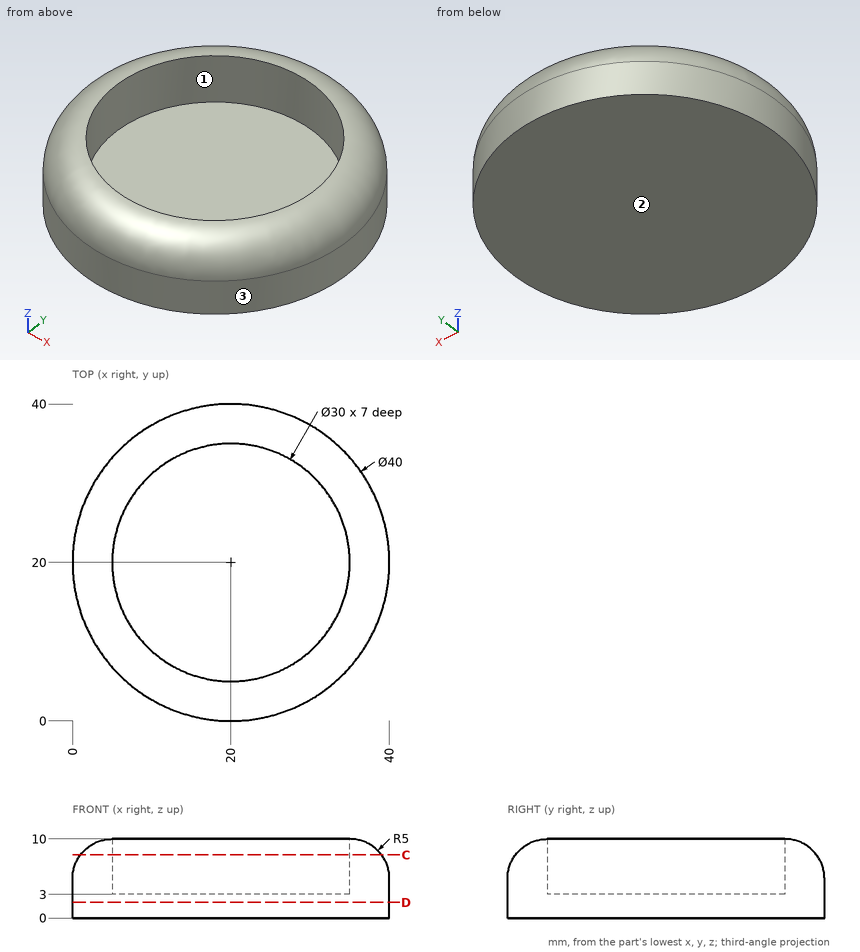
Design review of the part shown in the three views and the two pictorial views. Dimensions are in mm from the part's minimum x, y and z. Give positions to 0.01 mm unless a question says otherwise; leave off trailing zeros. Loops run counter-clockwise (first coordinate to the right, second up) from the corner with the lowest first, then second, coordinate; pieces in that order, holes last. Notation, with made-up numbers: (74.25, 55) -> (89.25, 55) arc R31 cw to (89.25, 85) -> close; hole circle Ø8 at (7.5, -25.75). An arc over 180 degrees is marked (long way). One line per question, with ' | ' between items.
1) To check wall thickness, follow probe 1 along Y at (x, z) = (20, 5); probe 2 along Z at (x, y) = (23, 32.5); probe 3 along Y at (x, z) = (20, 6.5). State the ranges of each line that lie inside material, in increasing order.
Resolved:
probe 1: y = 0 to 5, 35 to 40 | probe 2: z = 0 to 3 | probe 3: y = 0.23 to 5, 35 to 39.77
2) The part is to be moulded in two halves that separate along Y. For the marked faces 1, 2 and 3, say which applies: +Y half, -Y half, draft (parallel to the pull), parting line (faces both ways), or undercut.
Resolved:
face 1: undercut | face 2: draft | face 3: parting line
3) We need section C-C (z = 8). Write out the cut boundary in (x, y).
Resolved:
outline: circle Ø38 at (20, 20); hole circle Ø30 at (20, 20)
4) We need section D-D (z = 2). Write out the cut boundary in (x, y).
Resolved:
outline: circle Ø40 at (20, 20)
5) Insertion check: pin 1 Ø1 at (x, z) = (17, 7) entering from -Y; pin 2 Ø2 at (x, y) = (34.5, 32.5) entering from +Z; pin 3 Ø5 at (x, z) = (7, 4.5) entering from -Y. Each pin has a flat end and moves straight along its axis. Give the tip position at first contact, or say it passes through.
Resolved:
pin 1: stops at y = 0.44 | pin 2: stops at z = 8.89 | pin 3: stops at y = 2.98
